Geometry: final body of the model. Coordinates: model frame, mm. A direction names the side the tool comes from. Give positions to 0.01 mm unless a question says otherwise; leave off trailing zeros. Loops run counter-clockwise (first coordinate to the right, second up) from the corner with the lowest first, then second, coordinate; pieces in that order, holes last.
1. Access query for faces 5 (the face through (17.5, -21, 28)), 6 (the face through (18.98, 17.22, 18.13)), 7 (the face through (10, 13.5, 2)). Directions: +Z, -Z, +X, -X, +Y, -Y. A direction counts if a zero-diameter tool reaches every point of the face in a straight line with its end or side. Return the directions, or none.
2. Material intervals for line 1 along Z through (x, y) = (-3.5, 8); line 2 along X through (y, z) = (-30, 36); line 3 along Y through (x, z) = (18, 45), sorted ascending.
3. Section D-D, the plane z = 18.75. Output: boundary loops of the cut face in (x, y), then the cut area to 3 significant figures.
4. Draft query along X for faces 1 (the face through (0, 0, 3)), 2 (the face through (6.2, -8.04, 1.52)), 3 (the face through (16.64, 0.19, 3.9)), 4 (the face through (18.789, 0.189, 1.804)). Return one class per face: +X half, -X half, draft (parallel to the pull), parting line (faces both ways), or undercut.
5. Section C-C, the plane y = 3. Output: boundary loops of the cut face in (x, z).
6. First-contact query: P1, Ø8, axis at x = -5, y = -0.5, coming from the +Z side; P2, Ø4.5, axis at y = 16.02, z = 18.75, coming from the -X side; P3, Ø5, axis at x = 6.5, z = 2, coming from the -Y side. Flat tips, straight axial feed; report the tip coordinate or a pass-through.
7. Section A-A, the plane x = 5. Output: boundary loops of the cut face in (y, z).
8. Section B-B, the plane y = -45. Output: boundary loops of the cut face in (x, z).
Autodesk Inventor part; units mm, degrees
ref_plane "YZ Plane" through (0, 0, 0) normal (1, 0, 0) x (0, 1, 0)
ref_plane "XZ Plane" through (0, 0, 0) normal (0, 1, 0) x (-1, 0, 0)
ref_plane "XY Plane" through (0, 0, 0) normal (0, 0, 1) x (1, 0, 0)
sketch "スケッチ1" plane through (0, 0, 0) normal (0, 0, 1) x (1, 0, 0)
  circle A0 centre (0, 0) radius 13.5
  line L0 (0, 13.5) -> (14.5, 13.5)
  line L1 (14.5, 13.5) -> (14.5, -13.5)
  line L2 (14.5, -13.5) -> (0, -13.5)
  line L3 (0, -13.5) -> (0, 13.5)
  line L4 (0, 0) -> (14.5, 0) construction
  point P0 (0, 13.5)
  point P1 (0, -13.5)
  point P2 (0, -13.5)
  dimension "d0" = 27
  dimension "d1" = 27
  dimension "d2" = 14.5
extrude "プレート1" add sketch "スケッチ1" along normal blind 3
sketch "スケッチ2" plane through (17.5, 13.5, 6) normal (1, 0, 0) x (0, 1, 0)
  line L0 (-27, 0) -> (0, 0)
  line L1 (0, 0) -> (0, 19)
  line L2 (0, 19) -> (-27, 19)
  line L3 (-27, 19) -> (-27, 0)
edge flange "フランジ1" height 25 angle 90 thickness 3 bend radius 3 thickness toward (1, 0, 0) relief tear relief width 3 relief depth 1.5 edges at (14.5, 0, 3) wall of the first edge with corners at (17.5, -13.5, 6) (17.5, 13.5, 6) (17.5, 13.5, 25) (17.5, -13.5, 25)
bend "曲げ1"
corner "コーナー1"
sketch "スケッチ3" plane through (0, 0, 0) normal (0, 0, -1) x (-1, 0, 0)
  point P0 (0, 0)
  point P1 (10, 0)
  point P2 (-5, 8.6603)
  point P3 (-5, -8.6603)
  dimension "d14" = 10
  dimension "d17" = 360
hole "穴1" at (-10, 0, 0) at (5, 8.6603, 0) at (5, -8.6603, 0) direction (0, 0, 1) diameter 2.7 depth 3
sketch "スケッチ4" plane through (20.5, -13.5, 25) normal (1, 0, 0) x (0, 0, -1)
  circle A0 centre (-3, 13.5) radius 22
  line L0 (25, 27) -> (25, 0)
  line L1 (0, 27) -> (19, 27)
  point P0 (25, 13.5)
  dimension "d26" = 44
  dimension "d29" = 28
  dimension "d62" = 13.5
extrude "押し出し1" add sketch "スケッチ4" against normal up to surface (3 mm away)
sketch "スケッチ5" plane through (20.5, -13.5, 6) normal (1, 0, 0) x (0, 0, -1)
  arc A0 (-4.629, 27) -> (-4.629, 0) centre (-22, 13.5) ccw
  circle A1 centre (-22, 13.5) radius 14.5
  point P0 (6, 13.5)
  dimension "d30" = 29
extrude "押し出し2" cut sketch "スケッチ5" against normal up to surface (3 mm away)
sketch "スケッチ6" plane through (20.5, 0, 28) normal (1, 0, 0) x (0, 0, 1)
  point P0 (-28, 0)
sketch "スケッチ7" plane through (20.5, -13.5, 6) normal (1, 0, 0) x (0, 0, -1)
  circle A0 centre (-22, 13.5) radius 14.5
  point P0 (6, 13.5)
  point P1 (-40.5, 13.5)
  point P2 (-12.75, -2.5215)
  point P3 (-12.75, 29.5215)
  dimension "d33" = 18.5
  dimension "d36" = 360
hole "穴2" at (20.5, 0, 46.5) at (20.5, -16.0215, 18.75) at (20.5, 16.0215, 18.75) direction (-1, 0, 0) diameter 2.7 depth 3
fillet "フィレット1" radius 10 2 edges at (19, 13.5, 10.629) (19, -13.5, 10.629)
sketch "スケッチ8" plane through (20.5, -13.5, 6) normal (1, 0, 0) x (0, 0, -1)
  arc A0 (-7.0676, 29.6563) -> (-7.0676, -2.6562) centre (-22, 13.5) ccw
  line L0 (-44, 13.5) -> (-7, 13.5)
  line L1 (-7, 13.5) -> (-7, -36.5)
  line L2 (-7, -36.5) -> (-44, -36.5)
  line L3 (-44, -36.5) -> (-44, 13.5)
  arc A1 (-7.0676, 29.6562) -> (-0.2802, 27) centre (-0.2802, 37) ccw
  line L4 (0, 0) -> (0, 27)
  line L5 (0, 0) -> (-0.2802, 0)
  arc A2 (-0.2802, 0) -> (-7.0676, -2.6562) centre (-0.2802, -10) ccw
  arc A3 (-7.0676, 29.6562) -> (-7.0676, -2.6562) centre (-22, 13.5) ccw
  circle A4 centre (-12.75, 29.5215) radius 1.35
  circle A5 centre (-12.75, -2.5215) radius 1.35
  circle A6 centre (-22, 13.5) radius 14.5
  circle A7 centre (-40.5, 13.5) radius 1.35
  point P0 (6, 13.5)
  point P1 (-11.4, 29.5215)
  point P2 (-11.4, 29.5215)
  point P3 (-11.4, -2.5215)
  point P4 (-11.4, -2.5215)
  point P5 (-7.5, 13.5)
  point P6 (-7.5, 13.5)
  point P7 (-39.15, 13.5)
  point P8 (-39.15, 13.5)
  point P9 (-7, -2.5943)
  point P10 (-7.0676, -2.6562)
  dimension "d46" = 50
  dimension "d47" = 37
extrude "押し出し3" add sketch "スケッチ8" against normal up to surface (3 mm away) contours A0 A2 L1 L2 L3
fillet "フィレット2" radius 4 1 edges at (19, -16.0943, 13)
fillet "フィレット3" radius 4 2 edges at (19, -50, 13) (19, -50, 50)
sketch "スケッチ9" plane through (20.5, -13.5, 6) normal (1, 0, 0) x (0, 0, -1)
  line L0 (-44, 13.5) -> (-44, -32.5)
  line L1 (-44, -31.5) -> (-6.9219, -31.5) construction
  line L2 (-40, -36.5) -> (-11, -36.5)
  line L3 (-7, -32.5) -> (-7, -4.6519)
  point P0 (6, 13.5)
  point P1 (-39, -31.5)
  point P2 (-12, -31.5)
  dimension "d52" = 5
  dimension "d53" = 5
  dimension "d54" = 5
hole "穴3" at (20.5, -45, 45) at (20.5, -45, 18) direction (-1, 0, 0) diameter 4.2 depth 3
equation "\"d24\" = Thickness"
equation "\"d60\" = Thickness"
equation "\"d3\" = Thickness"
equation "\"d4\" = BendReliefWidth"
equation "\"d5\" = BendReliefDepth"
equation "\"d6\" = MinimumRemnant"
equation "\"d7\" = TransitionRadius"
equation "\"d10\" = BendRadius"
equation "\"d11\" = CornerReliefSize"
equation "\"d12\" = GapSize"
equation "\"d13\" = JacobiRadiusSize"
equation "\"BendRadius\" = Thickness"
equation "\"BendReliefWidth\" = Thickness"
equation "\"BendReliefDepth\" = 0.5 * Thickness"
equation "\"CornerReliefSize\" = 4 * Thickness"
equation "\"MinimumRemnant\" = 2 * Thickness"
equation "\"TransitionRadius\" = BendRadius"
equation "\"JacobiRadiusSize\" = BendRadius"
equation "\"GapSize\" = Thickness"
properties part number "hand_plate" material "アルミニウム 6061"
Answers below:
1. face 5: +Z, -X, +Y, -Y
1. face 6: +X, -X
1. face 7: -Z, +X, -X, +Y
2. line 1: z = 0 to 3
2. line 2: x = 17.5 to 20.5
2. line 3: y = -50 to -47.1, -42.9 to 13.96
3. outline: (17.5, -50) - (20.5, -50) - (20.5, -46.96) - (17.5, -46.96) - close; (17.5, -43.04) - (20.5, -43.04) - (20.5, -17.37) - (17.5, -17.37) - close; (17.5, -14.67) - (20.5, -14.67) - (20.5, -11.17) - (17.5, -11.17) - close; (17.5, 11.17) - (20.5, 11.17) - (20.5, 14.67) - (17.5, 14.67) - close; (17.5, 17.37) - (20.5, 17.37) - (20.5, 19.96) - (17.5, 19.96) - close
3. area: 115 mm2
4. face 1: draft
4. face 2: undercut
4. face 3: -X half
4. face 4: +X half
5. outline: (-13.16, 0) - (14.5, 0) arc R6 ccw to (20.5, 6) - (20.5, 13.81) - (17.5, 13.81) - (17.5, 6) arc R3 cw to (14.5, 3) - (-13.16, 3) - close; (17.5, 42.19) - (20.5, 42.19) - (20.5, 49.79) - (17.5, 49.79) - close
6. P1: stops at z = 3
6. P2: stops at x = 17.5
6. P3: stops at y = -13.5
7. outline: (-13.5, 0) - (-10.01, 0) - (-10.01, 3) - (-13.5, 3) - close; (-7.31, 0) - (7.31, 0) - (7.31, 3) - (-7.31, 3) - close; (10.01, 0) - (13.5, 0) - (13.5, 3) - (10.01, 3) - close
8. outline: (17.5, 13) - (20.5, 13) - (20.5, 15.9) - (17.5, 15.9) - close; (17.5, 20.1) - (20.5, 20.1) - (20.5, 42.9) - (17.5, 42.9) - close; (17.5, 47.1) - (20.5, 47.1) - (20.5, 50) - (17.5, 50) - close
